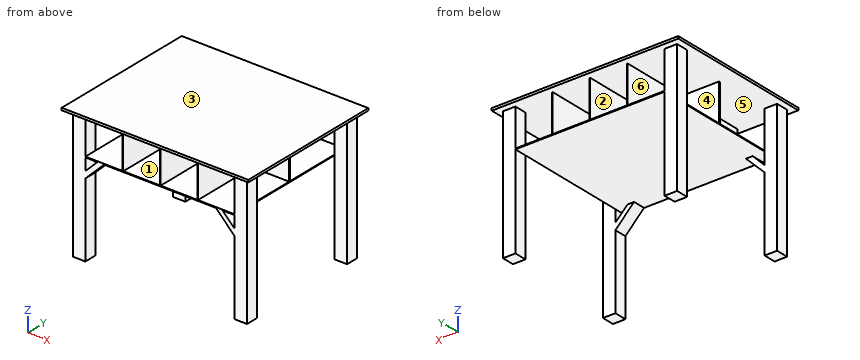
```python
from build123d import *

# Parameters (mm, degrees)
F0_W      = 1524
F0_H      = 1219.2
F1_DEPTH  = 19.05
F2_W      = 101.6
F2_H      = 101.6
F3_DEPTH  = 1066.8
F4_W      = 101.6
F4_H      = 6.35
F5_DEPTH  = 1219.2
F6_W      = 1219.2
F6_H      = 6.35
F7_DEPTH  = 1016
F8_W      = 1219.2
F8_H      = 9.5504
F9_DEPTH  = 311.658
F10_W     = 4.7752
F10_H     = 304.8
F11_DEPTH = 554.482
F12_DEPTH = 563.118
F14_DEPTH = 101.6
F15_DEPTH = 101.6


with BuildPart() as f1:
    # F0 (on Top) → F1 (new body)
    with BuildSketch(Plane.XY):
        with Locations((-82.5799548888, -2.5221072137)):
            Rectangle(F0_W, F0_H)
    extrude(amount=F1_DEPTH)

    # F2 (on face) → F3 (join)
    with BuildSketch(Plane.XY):
        with Locations((-742.9799548888, -510.5221072137)):
            Rectangle(F2_W, F2_H)
        with Locations((577.8200451112, -510.5221072137)):
            Rectangle(F2_W, F2_H)
        with Locations((577.8200451112, 505.4778927863)):
            Rectangle(F2_W, F2_H)
        with Locations((-742.9799548888, 505.4778927863)):
            Rectangle(F2_W, F2_H)
    extrude(amount=-F3_DEPTH)

    # F4 (on face) → F5 (join, through all)
    with BuildSketch(Plane.YZ.offset(-692.1799548888)):
        with Locations((-510.5221072137, -307.975)):
            Rectangle(F4_W, F4_H)
    extrude(amount=F5_DEPTH)

    # F6 (on face) → F7 (join)
    with BuildSketch(Plane(origin=(0, -459.7221072137, 0), x_dir=(-1, 0, 0), z_dir=(0, 1, 0))):
        with Locations((82.5799548888, -307.975)):
            Rectangle(F6_W, F6_H)
    extrude(amount=F7_DEPTH)

    # F8 (on face) → F9 (join)
    with BuildSketch(Plane(origin=(0, 0, -311.15), x_dir=(1, 0, 0), z_dir=(0, 0, -1))):
        with Locations((-82.5799548888, 2.5221072137)):
            Rectangle(F8_W, F8_H)
    extrude(amount=-F9_DEPTH)

    # F10 (on face) → F11 (join)
    with BuildSketch(Plane.XZ.offset(7.2973072137)):
        with Locations((-384.9923548888, -152.4)):
            Rectangle(F10_W, F10_H)
        with Locations((-80.1923548888, -152.4)):
            Rectangle(F10_W, F10_H)
        with Locations((224.6076451112, -152.4)):
            Rectangle(F10_W, F10_H)
    extrude(amount=F11_DEPTH)

    # F10 (on face) → F12 (join)
    with BuildSketch(Plane.XZ.offset(7.2973072137)):
        with Locations((-384.9923548888, -152.4)):
            Rectangle(F10_W, F10_H)
        with Locations((-80.1923548888, -152.4)):
            Rectangle(F10_W, F10_H)
        with Locations((224.6076451112, -152.4)):
            Rectangle(F10_W, F10_H)
    extrude(amount=-F12_DEPTH)

    # F13 (on face) → F14 (join)
    with BuildSketch(Plane.XZ.offset(561.3221072137)):
        Polygon((-692.1799548888, -409.6684632736), (-692.1799548888, -463.55), (-539.7799548888, -311.15), (-593.6614916152, -311.15), align=None)
    extrude(amount=-F14_DEPTH)

    # F13 (on face) → F15 (join)
    with BuildSketch(Plane.XZ.offset(561.3221072137)):
        Polygon((428.2372277794, -311.15), (374.355691053, -311.15), (527.0200451112, -463.8143540582), (527.0200451112, -409.9328173318), align=None)
    extrude(amount=-F15_DEPTH)


solid = f1.part
```
Here's how the part is built. I have some questions about the finished solid (model axes, mm). Face numbers are marked on the shaded views. A direction names the side the tool comes from. Round coordinates to 2 decimals unless told otherwise and drop trailing zeros. Order: outer loops, then holes, each group sorted by start corner. A loop starts at its lowest first (then second) coordinate and runs counter-clockwise, first axis right, second up. Notation, with made-up numbers: (59.25, -33.5) -> (69.25, -33.5) arc R17 cw to (69.25, -9.5) -> close; hole circle Ø5 at (58.5, 87.25). An arc over 180 degrees is marked (long way). Use a Markdown table: item, result. Add a question column.
(1) I need wall thicknesses on line 1 along X through (y, z) = (275, -157); line 2 along Z through (x, y) = (-171, 492); line 3 along X through (y, z) = (-473, -648.5). Which ranges of each line are inside material? Lowest first, please.
(2) Suppose I cut it at B-B, the plane z = -689. Please give me the cut outline in (x, y).
(3) If we mould it in two halves opening along Y, with no side actions, what happens to the marked faces 4, 5 and 6? For each: released by +Y, released by -Y, zero draft, split by the parting line, or undercut.
(4) For the marked faces 1, 2 and 3, which set-ups out of +Z, -Z, +X, -X, +Y, -Y let a thin tool reach every point of the face, with its end or its side?
(5) Suppose I cut it at A-A, the plane y = -142. Please give me the cut outline in (x, z).
(6) Suppose I cut it at C-C, the plane x = -450. Please give me the cut outline in (y, z).
(7) Suppose I cut it at D-D, the plane z = -357. Please give me the cut outline in (x, y), and give its area (3 significant figures).
(8) For pin 1 Ø2.5 at (x, z) = (224, -178) entering from -Y; pin 2 Ø10 at (x, z) = (-270, -173.5) entering from +Y; pin 3 Ø4 at (x, z) = (224.5, -129.5) entering from +Y, each with a flat end and sliding along its axis, tell me the tip position at first contact or that it passes through.
Verdict:
| question | item | result |
|---|---|---|
| 1 | line 1 | -387.38 to -382.6, -82.58 to -77.8, 222.22 to 227 |
| 1 | line 2 | -311.15 to -304.8, 0 to 19.05 |
| 1 | line 3 | -793.78 to -692.18, 527.02 to 628.62 |
| 2 | outline | (-793.78, -561.32) -> (-692.18, -561.32) -> (-692.18, -459.72) -> (-793.78, -459.72) -> close; (-793.78, 454.68) -> (-692.18, 454.68) -> (-692.18, 556.28) -> (-793.78, 556.28) -> close; (527.02, -561.32) -> (628.62, -561.32) -> (628.62, -459.72) -> (527.02, -459.72) -> close; (527.02, 454.68) -> (628.62, 454.68) -> (628.62, 556.28) -> (527.02, 556.28) -> close |
| 3 | face 4 | released by +Y |
| 3 | face 5 | undercut |
| 3 | face 6 | zero draft |
| 4 | face 1 | -Y |
| 4 | face 2 | +Y |
| 4 | face 3 | +Z, +X, -X, +Y, -Y |
| 5 | outline | (-844.58, 0) -> (-387.38, 0) -> (-387.38, -304.8) -> (-692.18, -304.8) -> (-692.18, -311.15) -> (527.02, -311.15) -> (527.02, -304.8) -> (227, -304.8) -> (227, 0) -> (679.42, 0) -> (679.42, 19.05) -> (-844.58, 19.05) -> close; hole (-382.6, -304.8) -> (-82.58, -304.8) -> (-82.58, 0) -> (-382.6, 0) -> close; hole (-77.8, -304.8) -> (222.22, -304.8) -> (222.22, 0) -> (-77.8, 0) -> close |
| 6 | outline | (-612.12, 0) -> (-7.3, 0) -> (-7.3, -304.8) -> (-561.32, -304.8) -> (-561.32, -311.15) -> (556.28, -311.15) -> (556.28, -304.8) -> (2.25, -304.8) -> (2.25, 0) -> (607.08, 0) -> (607.08, 19.05) -> (-612.12, 19.05) -> close |
| 7 | outline | (-793.78, -561.32) -> (-692.18, -561.32) -> (-692.18, -459.72) -> (-793.78, -459.72) -> close; (-793.78, 454.68) -> (-692.18, 454.68) -> (-692.18, 556.28) -> (-793.78, 556.28) -> close; (-639.51, -561.32) -> (-585.63, -561.32) -> (-585.63, -459.72) -> (-639.51, -459.72) -> close; (420.21, -561.32) -> (474.09, -561.32) -> (474.09, -459.72) -> (420.21, -459.72) -> close; (527.02, -561.32) -> (628.62, -561.32) -> (628.62, -459.72) -> (527.02, -459.72) -> close; (527.02, 454.68) -> (628.62, 454.68) -> (628.62, 556.28) -> (527.02, 556.28) -> close |
| 7 | area | 52,200 mm2 |
| 8 | pin 1 | y = -561.78 |
| 8 | pin 2 | y = 2.25 |
| 8 | pin 3 | y = 555.82 |
